Here's how the part is built. I have some questions about the finished solid (model axes, mm). Face numbers are marked on the shaded views. A direction names the side the tool comes from. Round coordinates to 2 decimals unless told otherwise and drop trailing zeros. Write each loop counter-clockwise with the first axis right and the second up, starting at its lowest first coordinate (ties: lowest second). Pieces come first, ordered by that corner, then holes. Notation, with made-up numbers: (-16, -22) - (-1, -22) arc R15 cw to (-1, -10) - close; hole circle Ø1 at (39.25, 13). An arc over 180 degrees is marked (long way). One line per question, with ' | ' between items. Start each with the question number.
(1) Imagine slicing it at B-B (x = 103). Write out the boundary of the cut face in (y, z).
(2) Thinking about a two-plate mould opening in X: for the marked faces 3, 4, 5 and 6, which applies, pulls with the +X half, pulls with the -X half, needs draft (parallel to the pull), parting line crosses it, or undercut?
(3) If I drill on L1, parallel to X at y = -13, z = 13; L2, parallel to Y at x = 112.95, z = 0; L3, parallel to X at y = -2, z = 8, over which ranges is the centre line in solid material (lowest first)?
(4) Will these pins go through, and if not, where does the flat tip stop? pin 1 (0.8 mm diameter, centred on y = -8, z = 12.5, fed in from +X); pin 2 (19 mm diameter, centred on y = 2.5, z = -9, fed in from -X); pin 3 (8 mm diameter, centred on x = 72.5, y = 11.5, fed in from +Z); pin 4 (1 mm diameter, centred on x = 27, y = 12, fed in from -Z) (3 decimals).
(5) Imagine slicing it at A-A (x = 42.5). Write out the boundary of the cut face in (y, z).
(6) For the marked faces 1 and 2, which set-ups out of +Z, -Z, +X, -X, +Y, -Y let a thin tool reach every point of the face, with its end or its side?
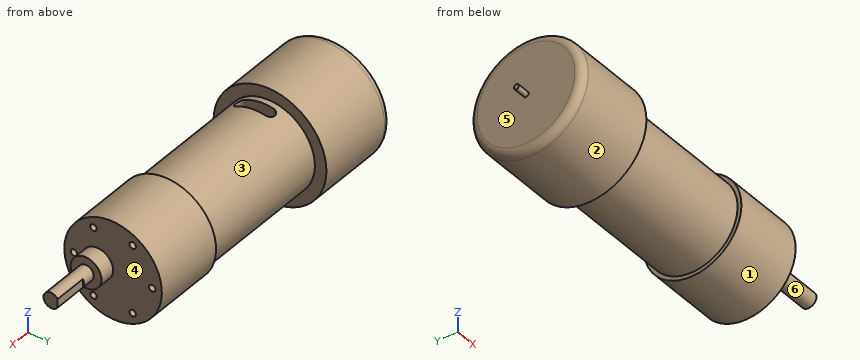
from build123d import *

# Parameters (mm, degrees)
SKETCH1_R           = 22
BOSS_EXTRUDE1_DEPTH = 33
SKETCH2_R           = 17.5
BOSS_EXTRUDE2_DEPTH = 53
SKETCH4_R           = 19
BOSS_EXTRUDE3_DEPTH = 28
CUT_EXTRUDE1_DEPTH  = 119.169369974
SKETCH13_R          = 1.25
CUT_EXTRUDE2_DEPTH  = 3.5
SKETCH15_R          = 6
BOSS_EXTRUDE4_DEPTH = 6
SKETCH16_R          = 3
BOSS_EXTRUDE5_DEPTH = 24
CUT_EXTRUDE3_DEPTH  = 13
FILLET1_R           = 3
SKETCH18_R          = 1
BOSS_EXTRUDE6_DEPTH = 5


with BuildPart() as part:
    # Sketch1 → Boss-Extrude1 (new body)
    with BuildSketch(Plane(origin=(0, 0, 0), x_dir=(0, 0, -1), z_dir=(1, 0, 0))):
        Circle(SKETCH1_R)
    extrude(amount=BOSS_EXTRUDE1_DEPTH)

    # Sketch2 → Boss-Extrude2 (add)
    with BuildSketch(Plane(origin=(33, 0, 0), x_dir=(0, 0, -1), z_dir=(1, 0, 0))):
        Circle(SKETCH2_R)
    extrude(amount=BOSS_EXTRUDE2_DEPTH)

    # Sketch4 → Boss-Extrude3 (add)
    with BuildSketch(Plane(origin=(86, 0, 0), x_dir=(0, 0, -1), z_dir=(1, 0, 0))):
        Circle(SKETCH4_R)
    extrude(amount=BOSS_EXTRUDE3_DEPTH)

    # Sketch12 → Cut-Extrude1 (cut, through all)
    with BuildSketch(Plane.XY):
        with BuildLine():
            Line((39.717889668, 3.156796221), (39.717889668, -7.930488068))
            ThreePointArc((39.717889668, -7.930488068), (37.562028834, -10.086348902), (35.406168, -7.930488068))
            Line((35.406168, -7.930488068), (35.406168, 3.156796221))
            ThreePointArc((35.406168, 3.156796221), (37.562028834, 5.312657055), (39.717889668, 3.156796221))
        make_face()
    extrude(amount=CUT_EXTRUDE1_DEPTH, mode=Mode.SUBTRACT)

    # Sketch13 → Cut-Extrude2 (cut)
    with BuildSketch(Plane(origin=(114, 0, 0), x_dir=(0, 0, -1), z_dir=(1, 0, 0))):
        with Locations((0, 15.25)):
            Circle(SKETCH13_R)
        with Locations((13.206887408, 7.625)):
            Circle(SKETCH13_R)
        with Locations((13.206887408, -7.625)):
            Circle(SKETCH13_R)
        with Locations((0, -15.25)):
            Circle(SKETCH13_R)
        with Locations((-13.206887408, -7.625)):
            Circle(SKETCH13_R)
        with Locations((-13.206887408, 7.625)):
            Circle(SKETCH13_R)
    extrude(amount=-CUT_EXTRUDE2_DEPTH, mode=Mode.SUBTRACT)

    # Sketch15 → Boss-Extrude4 (add)
    with BuildSketch(Plane(origin=(114, 0, 0), x_dir=(0, 0, -1), z_dir=(1, 0, 0))):
        with Locations((0, -6)):
            Circle(SKETCH15_R)
    extrude(amount=BOSS_EXTRUDE4_DEPTH)

    # Sketch16 → Boss-Extrude5 (add)
    with BuildSketch(Plane(origin=(114, 0, 0), x_dir=(0, 0, -1), z_dir=(1, 0, 0))):
        with Locations((0, -6)):
            Circle(SKETCH16_R)
    extrude(amount=BOSS_EXTRUDE5_DEPTH)

    # Sketch17 → Cut-Extrude3 (cut)
    with BuildSketch(Plane(origin=(138, 0, 0), x_dir=(0, 0, -1), z_dir=(1, 0, 0))):
        Polygon((1.658312395, -3.5), (3, -3.5), (3, -1.535610447), (1.658312395, -1.535610447), (-2.178415849, -1.535610447), (-2.178415849, -3.5), align=None)
    extrude(amount=-CUT_EXTRUDE3_DEPTH, mode=Mode.SUBTRACT)

    # Fillet1
    fillet1_edges = [part.edges().sort_by_distance(p)[0] for p in [
        (0, 0, 22),
    ]]
    fillet(fillet1_edges, radius=FILLET1_R)

    # Sketch18 → Boss-Extrude6 (add)
    with BuildSketch(Plane.ZY):
        with Locations(Location((0, 0, 0), (0, 0, 180))):
            Circle(SKETCH18_R)
    extrude(amount=BOSS_EXTRUDE6_DEPTH)


solid = part.part
Check sheet entries:
1) outline: circle Ø38 at (0, 0)
2) face 3: undercut | face 4: pulls with the +X half | face 5: pulls with the -X half | face 6: needs draft
3) L1: 0 to 33, 86 to 114 | L2: -19 to -16.5, -14 to 14, 16.5 to 19 | L3: 0 to 35.41, 39.72 to 114
4) pin 1: x = 110.5 | pin 2: x = -5 | pin 3: z = 15.81 | pin 4: z = -18.755
5) outline: circle Ø35 at (0, 0)
6) face 1: +X | face 2: +X, -X
